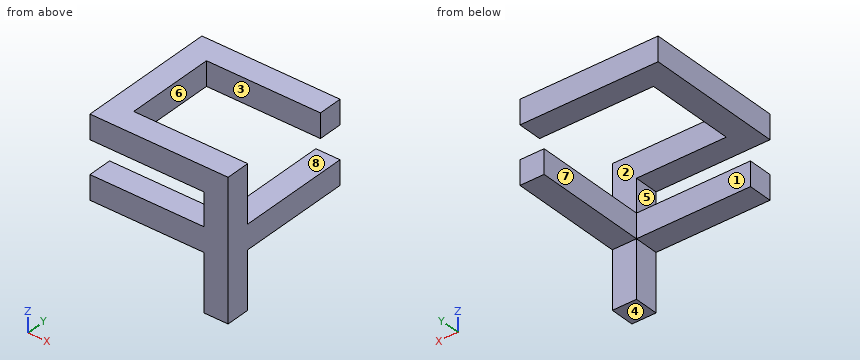
from build123d import *

# Parameters (mm, degrees)
F1_DEPTH = 177.8
F2_W     = 177.8
F2_H     = 241.3
F2_H_2   = 177.8
F2_H_3   = 419.1
F2_W_2   = 838.2
F3_DEPTH = 177.8
F4_W     = 838.2
F4_H     = 177.8
F5_DEPTH = 177.8


with BuildPart() as f1:
    # F0 (on Top) → F1 (new body)
    with BuildSketch(Plane.XY):
        Polygon((508, 330.2), (508, 508), (-508, 508), (-508, -508), (508, -508), (508, -330.2), (-330.2, -330.2), (-330.2, 330.2), align=None)
    extrude(amount=F1_DEPTH)

    # F2 (on face) → F3 (join)
    with BuildSketch(Plane.XZ.offset(508)):
        with Locations((419.1, -120.65)):
            Rectangle(F2_W, F2_H)
        with Locations((419.1, -330.2)):
            Rectangle(F2_W, F2_H_2)
        with Locations((419.1, -628.65)):
            Rectangle(F2_W, F2_H_3)
        with Locations((-88.9, -330.2)):
            Rectangle(F2_W_2, F2_H_2)
    extrude(amount=-F3_DEPTH)

    # F4 (on face) → F5 (join)
    with BuildSketch(Plane.YZ.offset(508)):
        with Locations((88.9, -330.2)):
            Rectangle(F4_W, F4_H)
    extrude(amount=-F5_DEPTH)


solid = f1.part
Design review of the part built by this model. Coordinates are the model's own, in mm. Face numbers are marked on the shaded views. A direction names the side the tool comes from. Coordinates: 2 decimals unless noted, no trailing zeros. Order: outer loops, then holes, each group sorted by start corner. A loop starts at its lowest first (then second) coordinate and runs counter-clockwise, first axis right, second up.
Item 1: Take a section at A-A, the plane x = 17.5. Write out the cut boundary in (y, z).
Item 2: The part is to be moulded in two halves that separate along Y. For the marked faces 1, 2, 3 and 4, say which applies: pulls with the +Y half, pulls with the -Y half, needs draft (parallel to the pull), parting line crosses it, or undercut.
Item 3: Take a section at C-C, the plane x = -417.5. Write out the cut boundary in (y, z).
Item 4: Take a section at B-B, the plane y = 138. Write out the cut boundary in (x, z).
Item 5: For line 1 (Y direction, x = -75, z = 8.5); line 2 (Z direction, x = -467, y = 58); line 3 (Y direction, x = 419, z = -785), list the stretches that pass through material, from the lowest coordinate up.
Item 6: For the marked faces 5, 6, 7 and 8, list the 3-axis set-ups (+Z, -Z, +X, -X, +Y, -Y) from which the entire face can be reached by the end or side of a thin tool; tool diameter is ignored.
Item 7: Take a section at D-D, the plane y = -422.5. Write out the cut boundary in (x, z), then the cut area to 3 significant figures.
The answers:
1. outline: (-508, -419.1) - (-330.2, -419.1) - (-330.2, -241.3) - (-508, -241.3) - close; (-508, 0) - (-330.2, 0) - (-330.2, 177.8) - (-508, 177.8) - close; (330.2, 0) - (508, 0) - (508, 177.8) - (330.2, 177.8) - close
2. face 1: pulls with the +Y half
2. face 2: undercut
2. face 3: undercut
2. face 4: needs draft
3. outline: (-508, -419.1) - (-330.2, -419.1) - (-330.2, -241.3) - (-508, -241.3) - close; (-508, 0) - (508, 0) - (508, 177.8) - (-508, 177.8) - close
4. outline: (-508, 0) - (-330.2, 0) - (-330.2, 177.8) - (-508, 177.8) - close; (330.2, -419.1) - (508, -419.1) - (508, -241.3) - (330.2, -241.3) - close
5. line 1: y = -508 to -330.2, 330.2 to 508
5. line 2: z = 0 to 177.8
5. line 3: y = -508 to -330.2
6. face 5: -X, +Y, -Y
6. face 6: +Z, -Z, +X
6. face 7: -Z, -X, +Y
6. face 8: +X, -X, +Y
7. outline: (-508, -419.1) - (330.2, -419.1) - (330.2, -838.2) - (508, -838.2) - (508, 177.8) - (-508, 177.8) - (-508, 0) - (330.2, 0) - (330.2, -241.3) - (-508, -241.3) - close
7. area: 479,000 mm2
